The drawing under review shows one solid part. Ordinate dimensions are in mm from its lowest x, y, z. Round coordinates to 2 decimals unless told otherwise and drop trailing zeros. Write each loop counter-clockwise with the first axis right and the second up, starting at its lowest first coordinate (ties: lowest second). Pieces come first, ordered by that corner, then holes. Notation, with made-up numbers: (85.25, -4.5) -> (95.25, -4.5) arc R23 cw to (95.25, 16.5) -> close; hole circle Ø1 at (-27, -16). An arc over 180 degrees is marked (long way). Answer in a Markdown table with one row per item.
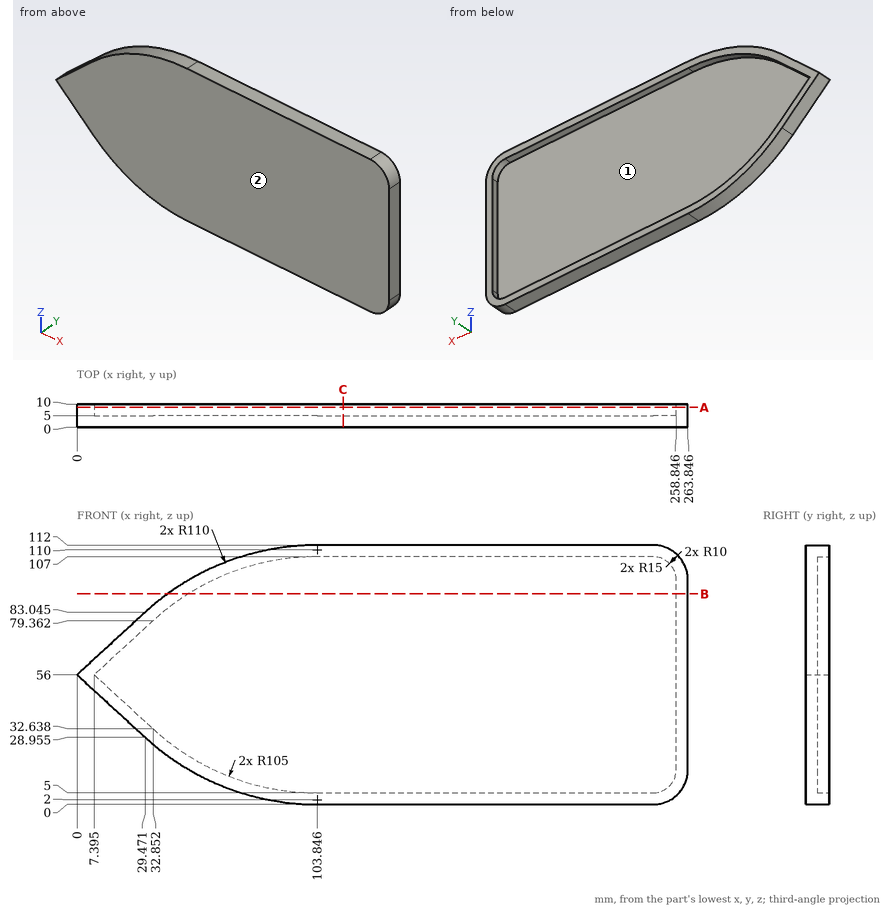
1) Consider section B-B on z = 91. State the section outline as (x, y) points, then the cut area to 3 significant figures.
Solved:
| item | result |
|---|---|
| outline | (39.2, 0) -> (263.85, 0) -> (263.85, 10) -> (258.85, 10) -> (258.85, 5) -> (48.13, 5) -> (48.13, 10) -> (39.2, 10) -> close |
| area | 1,190 mm² |
2) Consider section A-A on y = 8.5. State the section outline as (x, z) points (1 decimal), then the cut area to 3 significant figures.
Solved:
| item | result |
|---|---|
| outline | (0, 56) -> (29.5, 29) arc R110 ccw to (103.8, 0) -> (248.8, 0) arc R15 ccw to (263.8, 15) -> (263.8, 97) arc R15 ccw to (248.8, 112) -> (103.8, 112) arc R110 ccw to (29.5, 83) -> close; hole (7.4, 56) -> (32.9, 32.6) arc R105 ccw to (103.8, 5) -> (248.8, 5) arc R10 ccw to (258.8, 15) -> (258.8, 97) arc R10 ccw to (248.8, 107) -> (103.8, 107) arc R105 ccw to (32.9, 79.4) -> close |
| area | 3,230 mm² |
3) Mouldability with a two-part tool opening along X and no side actions: class the marked faces 1 and 2 as pulls with the +X half, pulls with the -X half, needs draft (parallel to the pull), parting line crosses it, or undercut.
Solved:
| item | result |
|---|---|
| face 1 | undercut |
| face 2 | needs draft |
4) Clearance check with flat-ended pins moving along their axes: pin 1 Ø1.5 at (y, z) = (4, 74.5) entering from -X; pin 2 Ø6 at (x, z) = (43.5, 68.5) entering from +Y; pin 3 Ø6 at (x, y) = (47.5, 3.5) entering from -Z. State where each tip first meets the part, or that it passes through.
Solved:
| item | result |
|---|---|
| pin 1 | x = 19.34 |
| pin 2 | y = 5 |
| pin 3 | z = 13.8 |
5) Consider section C-C on x = 115. State the section outline as (y, z) points, then the cut area to 3 significant figures.
Solved:
| item | result |
|---|---|
| outline | (0, 0) -> (10, 0) -> (10, 5) -> (5, 5) -> (5, 107) -> (10, 107) -> (10, 112) -> (0, 112) -> close |
| area | 610 mm² |
6) For line 1 (Z direction, x = 241, y = 8.25); line 2 (Y direction, x = 125, z = 97); line 3 (X direction, y = 7.75, z = 31) (1 decimal), list the stretches that pass through material, from the lowest coordinate up. Write a range as [from, to].
Solved:
| item | result |
|---|---|
| line 1 | [0, 5], [107, 112] |
| line 2 | [0, 5] |
| line 3 | [27.2, 34.7], [258.8, 263.8] |
